Check sheet for the modelled part. Datum: model origin and axes. Units: mm. A direction names the side the tool comes from. Give positions to 0.01 mm unless a question says otherwise; leave off trailing zeros. Order: outer loops, then holes, each group sorted by start corner. A loop starts at its lowest first (then second) coordinate and runs counter-clockwise, first axis right, second up.
Item 1: Release check for a two-part mould opening along Y. For faces 5 (the flat face through (-49.019, -6, 16)), 6 (the flat face through (-36.344, 18.174, -14.949)), 7 (the flat face through (-25.03, -18.94, 16.16)), 8 (the cylindrical face through (-36.479, -8.612, 16.163)) record: released by +Y, released by -Y, zero draft, split by the parting line, or undercut.
Item 2: Sectioned sample at D-D on x = -35.5. Record the boundary of the cut face in (y, z), and give its area (3 significant figures).
Item 3: Material ranges on line 1 along Z through (x, y) = (-37, 1); line 2 along X through (y, z) = (13.75, 0); line 3 along X through (y, z) = (20, -2), recorded low to high.
Item 4: Access from +Z, -Z, +X, -X, +Y, -Y to the whole of each face (thin tool, end or side, straight path). Record for faces 1 (the cylindrical face through (-16, 16, -21)), 2 (the flat face through (15.16, 14.79, 18.7)), 3 (the flat face through (-20.882, 15, 0)), 4 (the flat face through (-24.019, -12, -16)).
Item 5: Sectioned sample at B-B on y = 4.5. Record the boundary of the cut face in (x, z).
Item 6: Gauge pin test, flat ends, axial feed: P1, Ø1, axis at y = 10.5, z = -6, coming from the -X side; P2, Ø1, axis at x = -10.5, z = -18, coming from the -Y side; P3, Ø6.5, axis at x = -37, y = -12.58, coming from the +Z side; P4, Ø1, axis at x = -35.5, z = 11, coming from the +Y side. Record the tip position at first contact, or that the pin passes through.
Item 7: Sectioned sample at A-A on x = 0. Record the boundary of the cut face in (y, z).
Item 8: Sectioned sample at C-C on z = 9. Record the boundary of the cut face in (x, y), and give its area (3 significant figures).
from build123d import *

# Parameters (mm, degrees)
EXTRUDE_1_DEPTH       = 30
SKETCH_2_R            = 15
CUT_EXTRUDE_2_DEPTH   = 45.532745299
EXTRUDE_3_DEPTH       = 45
CUT_EXTRUDE_START     = 70
SKETCH_3_W            = 44.656689001
SKETCH_3_H            = 20
CUT_EXTRUDE_1_DEPTH   = 130
SKETCH_7_R            = 3.999999997
CUT_EXTRUDE_2_2_DEPTH = 73.992250074
FILLET_1_R            = 5
CHAMFER_5_SIZE        = 2
SKETCH_10_R           = 17
CUT_EXTRUDE_5_DEPTH   = 3.5


with BuildPart() as part:
    # Эскиз1 → Вытянуть1 (new body)
    with BuildSketch(Plane(origin=(0, 0, 0), x_dir=(1, 0, 0), z_dir=(0, 1, 0))):
        Polygon((-24.019063342, 22.5), (10.980936658, 22.5), (19.22346273, 15), (19.22346273, -15), (10.980936658, -22.5), (-24.019063342, -22.5), align=None)
    extrude(amount=EXTRUDE_1_DEPTH)

    # Эскиз2 → Cut-Extrude 2 (cut, through all)
    with BuildSketch(Plane(origin=(0, 30, 0), x_dir=(1, 0, 0), z_dir=(0, 1, 0))):
        with Locations(Location((0, 0, 0), (0, 0, 270))):
            Circle(SKETCH_2_R)
    extrude(amount=-CUT_EXTRUDE_2_DEPTH, mode=Mode.SUBTRACT)

    # Эскиз6 → Вытянуть3 (add)
    with BuildSketch(Plane(origin=(0, 0, -22.5), x_dir=(-1, 0, 0), z_dir=(0, 0, -1))):
        Polygon((24.019063342, -19.927530698), (24.019063342, 30), (49.019063342, 6.012561534), (49.019063342, -19.927530698), align=None)
    extrude(amount=-EXTRUDE_3_DEPTH)

    # Эскиз3 → Вырез-Вытянуть1 (cut)
    with BuildSketch(Plane(origin=(0, 30, 0), x_dir=(1, 0, 0), z_dir=(0, 1, 0)).offset(CUT_EXTRUDE_START)):
        with Locations((-43.210774099, 0)):
            Rectangle(SKETCH_3_W, SKETCH_3_H)
    extrude(amount=-CUT_EXTRUDE_1_DEPTH, mode=Mode.SUBTRACT)

    # Эскиз7 → Cut-Extrude 2 2 (cut, through all)
    with BuildSketch(Plane(origin=(0, 0, -22.5), x_dir=(-1, 0, 0), z_dir=(0, 0, -1))):
        with Locations((37.000000002, -12.578306382)):
            Circle(SKETCH_7_R)
    extrude(amount=-CUT_EXTRUDE_2_2_DEPTH, mode=Mode.SUBTRACT)

    # Скругление1
    fillet_1_edges = [part.edges().sort_by_distance(p)[0] for p in [
        (-24.019063342, 0, -16.25),
    ]]
    fillet(fillet_1_edges, radius=FILLET_1_R)

    # Фаска5
    chamfer_5_edges = [part.edges().sort_by_distance(p)[0] for p in [
        (-49.019063342, -19.927530698, 16.25),
        (-24.019063342, -19.927530698, 16.25),
        (-24.019063342, -19.927530698, -16.25),
        (-49.019063342, -19.927530698, -16.25),
    ]]
    chamfer(chamfer_5_edges, length=CHAMFER_5_SIZE)

    # Эскиз10 → Вырез-Вытянуть5 (cut)
    with BuildSketch(Plane(origin=(0, 0, -22.5), x_dir=(-1, 0, 0), z_dir=(0, 0, -1))):
        with Locations((21.57600878, 32.059441466)):
            Circle(SKETCH_10_R)
    extrude(amount=-CUT_EXTRUDE_5_DEPTH, mode=Mode.SUBTRACT)


solid = part.part
Report:
1. face 5: zero draft
1. face 6: released by +Y
1. face 7: released by -Y
1. face 8: undercut
2. outline: (-19.93, -22.5) - (-16.29, -22.5) - (-16.29, -10) - (-19.93, -10) - close; (-19.93, 10) - (-16.29, 10) - (-16.29, 22.5) - (-19.93, 22.5) - close; (-8.87, -22.5) - (18.98, -22.5) - (18.98, -10) - (-8.87, -10) - close; (-8.87, 10) - (18.98, 10) - (18.98, 22.5) - (-8.87, 22.5) - close
2. area: 787 mm2
3. line 1: z = -22.5 to -10, 10 to 22.5
3. line 2: x = -20.88 to -15, 15 to 19.22
3. line 3: x = -20.88 to -14.87, 14.87 to 19.22
4. face 1: -Z, +Y
4. face 2: +Z, +X, +Y, -Y
4. face 3: -X, +Y, -Y
4. face 4: +Z, -Z, +X, -Y
5. outline: (-49.02, -22.5) - (10.98, -22.5) - (19.22, -15) - (19.22, 15) - (10.98, 22.5) - (-49.02, 22.5) - (-49.02, 10) - (-20.88, 10) - (-20.88, -10) - (-49.02, -10) - close; hole circle Ø30 at (0, 0)
6. P1: stops at x = -20.88
6. P2: stops at y = 0
6. P3: passes through
6. P4: stops at y = 19.46
7. outline: (0, -22.5) - (30, -22.5) - (30, -15) - (0, -15) - close; (0, 15) - (30, 15) - (30, 22.5) - (0, 22.5) - close
8. outline: (-20.88, -0.36) arc R5 cw to (-19.02, 0) - (-12, 0) - (-12, 30) - (-20.88, 30) - close; (12, 0) - (19.22, 0) - (19.22, 30) - (12, 30) - close
8. area: 483 mm2
